Autodesk Inventor part; units mm, degrees
ref_plane "YZ Plane" through (0, 0, 0) normal (1, 0, 0) x (0, 1, 0)
ref_plane "XZ Plane" through (0, 0, 0) normal (0, 1, 0) x (-1, 0, 0)
ref_plane "XY Plane" through (0, 0, 0) normal (0, 0, 1) x (1, 0, 0)
sketch "Sketch1" plane through (0, 0, 0) normal (0, 0, 1) x (1, 0, 0)
  line L0 (-210.6, 18) -> (39.4, 18)
  line L1 (39.4, 18) -> (39.4, -232)
  line L2 (39.4, -232) -> (-210.6, -232)
  line L3 (-210.6, -232) -> (-210.6, 18)
  line L4 (21.4, -214) -> (21.4, 0)
  line L5 (21.4, -214) -> (-192.6, -214)
  line L6 (-192.6, -214) -> (21.4, -214)
  line L7 (39.4, 0) -> (39.4, -21.4)
  line L8 (39.4, -21.4) -> (21.4, -21.4)
  line L9 (21.4, -21.4) -> (21.4, 0)
  line L10 (39.4, -64.2) -> (21.4, -64.2)
  line L11 (21.4, -64.2) -> (21.4, -85.6)
  line L12 (21.4, -85.6) -> (39.4, -85.6)
  line L13 (21.4, -128.4) -> (39.4, -128.4)
  line L14 (39.4, -149.8) -> (21.4, -149.8)
  line L15 (39.4, -192.6) -> (21.4, -192.6)
  line L16 (-210.6, 18) -> (-210.6, 0)
  line L17 (21.4, 0) -> (21.4, 18)
  line L18 (-210.6, -192.6) -> (-192.6, -192.6)
  line L19 (-210.6, -149.8) -> (-192.6, -149.8)
  line L20 (-192.6, -128.4) -> (-210.6, -128.4)
  line L21 (-192.6, -85.6) -> (-210.6, -85.6)
  line L22 (-210.6, -64.2) -> (-192.6, -64.2)
  line L23 (-210.6, -21.4) -> (-192.6, -21.4)
  line L24 (-64.2, -214) -> (-64.2, -232)
  line L25 (-107, -214) -> (-107, -232)
  line L26 (-128.4, -232) -> (-128.4, -214)
  line L27 (-171.2, -232) -> (-171.2, -214)
  line L28 (-42.8, -232) -> (-42.8, -214)
  line L29 (0, -232) -> (0, -214)
  line L30 (-64.2, 18) -> (-64.2, 0)
  line L31 (-42.8, 0) -> (-42.8, 18)
  line L32 (0, 0) -> (0, 18)
  line L33 (-128.4, 0) -> (-128.4, 18)
  line L34 (-171.2, 0) -> (-171.2, 18)
  line L35 (-107, 18) -> (-107, 0)
  line L36 (21.4, 0) -> (-192.6, 0)
  line L37 (-192.6, 0) -> (-192.6, -214)
  line L38 (21.4, -214) -> (21.4, -232)
  point P0 (0, 0)
  point P1 (227.0923, 209.5253)
  point P2 (245.0923, 209.5253)
  point P3 (227.0923, 252.3253)
  point P4 (205.6923, 273.7253)
  point P5 (205.6923, 291.7253)
  point P6 (162.8923, 291.7253)
  point P7 (162.8923, 273.7253)
  point P8 (141.4923, 273.7253)
  point P9 (141.4923, 291.7253)
  point P10 (98.6923, 291.7253)
  point P11 (98.6923, 273.7253)
  point P12 (77.2923, 273.7253)
  point P13 (77.2923, 291.7253)
  point P14 (34.4923, 291.7253)
  point P15 (34.4923, 273.7253)
  point P16 (13.0923, 252.3253)
  point P17 (-4.9077, 252.3253)
  point P18 (-4.9077, 209.5253)
  point P19 (13.0923, 209.5253)
  point P20 (13.0923, 188.1253)
  point P21 (-4.9077, 188.1253)
  point P22 (-4.9077, 145.3253)
  point P23 (13.0923, 145.3253)
  point P24 (13.0923, 123.9253)
  point P25 (-4.9077, 123.9253)
  point P26 (-4.9077, 81.1253)
  point P27 (13.0923, 81.1253)
  point P28 (13.0923, 59.7253)
  point P29 (34.4923, 59.7253)
  point P30 (34.4923, 41.7253)
  point P31 (77.2923, 41.7253)
  point P32 (77.2923, 59.7253)
  point P33 (98.6923, 59.7253)
  point P34 (98.6923, 41.7253)
  point P35 (141.4923, 41.7253)
  point P36 (141.4923, 59.7253)
  point P37 (162.8923, 59.7253)
  point P38 (162.8923, 41.7253)
  point P39 (205.6923, 41.7253)
  point P40 (205.6923, 59.7253)
  point P41 (227.0923, 59.7253)
  point P42 (227.0923, 81.1253)
  point P43 (245.0923, 81.1253)
  point P44 (245.0923, 123.9253)
  point P45 (227.0923, 123.9253)
  point P46 (227.0923, 145.3253)
  point P47 (245.0923, 145.3253)
  point P48 (245.0923, 188.1253)
  point P49 (227.0923, 188.1253)
  point P50 (-210.6, -232)
  dimension "d0" = 250
  dimension "d1" = 250
  dimension "d2" = 21.4
extrude "Plate1" add sketch "Sketch1" against normal blind 18 contours L0 L34 L36 L37 L23 L3 | L0 L35 L36 L33 | L36 L4 L5 L37 | L22 L37 L21 L3 | L0 L31 L36 L30 | L20 L37 L19 L3 | L0 L17 L36 L32 | L18 L37 L5 L27 L2 L3 | L10 L1 L12 L4 | L26 L5 L25 L2 | L13 L1 L14 L4 | L24 L5 L28 L2 | L29 L5 L38 L2
equation "\"d3\" = Thickness"
equation "\"BendRadius\" = Thickness"
equation "\"BendReliefWidth\" = Thickness"
equation "\"BendReliefDepth\" = 0.5 * Thickness"
equation "\"CornerReliefSize\" = 4 * Thickness"
equation "\"MinimumRemnant\" = 2 * Thickness"
equation "\"TransitionRadius\" = BendRadius"
equation "\"JacobiRadiusSize\" = BendRadius"
equation "\"GapSize\" = Thickness"
properties part number "6"
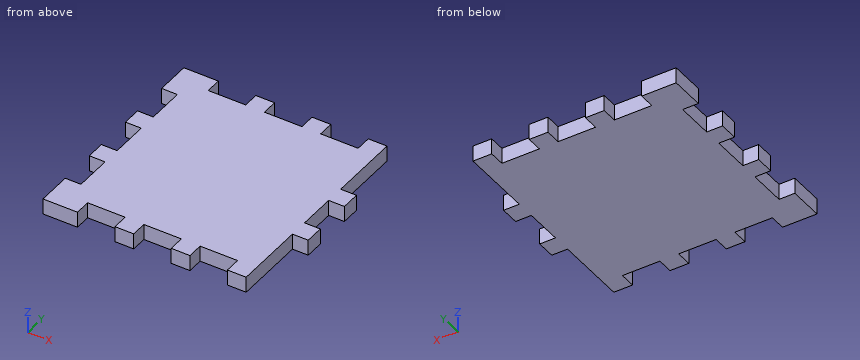
Design review of the part built by this model. Coordinates are the model's own, in mm. Give positions to 0.01 mm unless a question says otherwise; leave off trailing zeros. Order: outer loops, then holes, each group sorted by start corner. A loop starts at its lowest first (then second) coordinate and runs counter-clockwise, first axis right, second up. Notation, with made-up numbers: M -23.75,47.25 L 27.25,47.25 A30 cw 27.25,77.25 Z; hole C -32,60 d2. An arc over 180 degrees is marked long. One line per question, with ' | ' between items. Start each with the question number.
Q1. We need section A-A (x = -131.5). Write out the cut boundary in (y, z), plus the area to 3 significant figures.
Q2. For pin 1 Ø5.5 at (x, z) = (-157, -12) entering from -Y; pin 2 Ø6 at (y, z) = (-188, -14.5) entering from +X; pin 3 Ø5.5 at (x, z) = (31, -13) entering from -Y, all flat-tipped, find the tip position at first contact; note any pin that passes through.
Q3. For L1, parallel to Y at x = -198.5, z = -2; L2, parallel to Y at x = 23, z = -8; L3, parallel to X at y = -205, z = -9.5, list the stretches that pass through material, from the lowest coordinate up. Write a range as [from, to].
Q4. We need section B-B (y = -8). Write out the cut boundary in (x, z), plus the area to 3 significant figures.
Returned:
1) outline: M -214,-18 L 0,-18 L 0,0 L -214,0 Z | area: 3,850 mm2
2) pin 1: y = -214 | pin 2: x = 21.4 | pin 3: y = -149.8
3) L1: [-232, -192.6], [-149.8, -128.4], [-85.6, -64.2], [-21.4, 18] | L2: [-149.8, -128.4], [-85.6, -64.2] | L3: [-210.6, 21.4]
4) outline: M -210.6,-18 L 21.4,-18 L 21.4,0 L -210.6,0 Z | area: 4,180 mm2
